from build123d import *

# Parameters (mm, degrees)
F1_DEPTH = 25.4
F2_W     = 25.4
F2_H     = 37.8646999598
F3_DEPTH = 6.35
F5_DEPTH = 12.7
F7_DEPTH = 12.7


with BuildPart() as f1:
    # F0 (on Front) → F1 (new body)
    with BuildSketch(Plane.XZ):
        Polygon((-35.7808704906, 19.05), (-35.7808704906, 0), (-10.3808704906, 0), align=None)
    extrude(amount=F1_DEPTH)

    # F2 (on face) → F3 (join)
    with BuildSketch(Plane(origin=(0, 0, 0), x_dir=(1, 0, 0), z_dir=(0, 0, -1))):
        with Locations((-23.0808704906, 18.9323499799)):
            Rectangle(F2_W, F2_H)
    extrude(amount=F3_DEPTH)

    # F4 (on face) → F5 (cut)
    with BuildSketch(Plane.XZ.offset(25.4)):
        Polygon((-10.3808704906, 0), (-19.9058704906, 7.14375), (-19.9058704906, 0), align=None)
    extrude(amount=-F5_DEPTH, mode=Mode.SUBTRACT)

    # F6 (on face) → F7 (cut)
    with BuildSketch(Plane.XZ.offset(25.4)):
        Polygon((-35.7808704906, 19.05), (-35.7808704906, 12.7), (-27.3142038239, 12.7), align=None)
    extrude(amount=-F7_DEPTH, mode=Mode.SUBTRACT)


solid = f1.part
The listing builds one solid part. Answer for the finished solid, in the listing's coordinates (mm). A direction names the side the tool comes from. Coordinates: 2 decimals unless noted, no trailing zeros. Order: outer loops, then holes, each group sorted by start corner. A loop starts at its lowest first (then second) coordinate and runs counter-clockwise, first axis right, second up.
Q1. Given P1, Ø2, axis at x = -13.5, z = 4, coming from the -Y side; P2, Ø9.5, axis at x = -32.5, y = -16.5, coming from the +Z side; P3, Ø5.5, axis at y = -18, z = 2.5, coming from the +X side; P4, Ø1, axis at y = -7, z = 6, coming from the +X side, each flat-ended and moving along its own axis, determine where each tip first touches the part or whether it passes through.
Q2. A cutting plane is placed at C-C, the plane z = 1.75. Write down the section's boundary in (x, y), and give its area (3 significant figures).
Q3. A cutting plane is placed at A-A, the plane y = -24. Write down the section's boundary in (x, z), and give its area (3 significant figures).
Q4. A cutting plane is placed at D-D, the plane x = -18.5. Write down the section's boundary in (y, z).
Q5. Consider line 1 (Z direction, x = -17.75, y = -32); line 2 (X direction, y = -21.5, z = 3); line 3 (Z direction, x = -29.5, y = -16). Determine where each line is inside the solid, lowest interval first.
Q6. Which of the six approach directions +Z, -Z, +X, -X, +Y, -Y give full straight-line access (tool end or side, diameter ignored) to faces 1 (the face through (-26, 0, 4)), 2 (the face through (-33, -12.7, 15)), 3 (the face through (-19.906, -19, 4))?
Q7. A cutting plane is placed at B-B, the plane x = -30.25. Write down the section's boundary in (y, z), and give its area (3 significant figures).
Answers follow:
1. P1: passes through
1. P2: stops at z = 18.73
1. P3: stops at x = -10.38
1. P4: stops at x = -17.71
2. outline: (-35.78, -25.4) - (-19.91, -25.4) - (-19.91, -12.7) - (-12.71, -12.7) - (-12.71, 0) - (-35.78, 0) - close
2. area: 495 mm2
3. outline: (-35.78, -6.35) - (-10.38, -6.35) - (-10.38, 0) - (-19.91, 0) - (-19.91, 7.14) - (-27.31, 12.7) - (-35.78, 12.7) - close
3. area: 342 mm2
4. outline: (-37.86, -6.35) - (0, -6.35) - (0, 6.09) - (-12.7, 6.09) - (-12.7, 0) - (-37.86, 0) - close
5. line 1: z = -6.35 to 0
5. line 2: x = -35.78 to -19.91
5. line 3: z = -6.35 to 12.7
6. face 1: +Z, -Z, +X, -X, +Y
6. face 2: +Z, +X, -X, -Y
6. face 3: +Z, +X, -Y
7. outline: (-37.86, -6.35) - (0, -6.35) - (0, 14.9) - (-12.7, 14.9) - (-12.7, 12.7) - (-25.4, 12.7) - (-25.4, 0) - (-37.86, 0) - close
7. area: 591 mm2
